For this review, take the finished solid that the model builds, in its own axes (mm). A direction names the side the tool comes from. Give positions to 0.01 mm unless a question says otherwise; leave off trailing zeros. Loops run counter-clockwise (first coordinate to the right, second up) from the corner with the lowest first, then second, coordinate; pieces in that order, holes last. Notation, with made-up numbers: (-15, 43.5) - (43, 43.5) arc R11 cw to (43, 52.5) - close; hole circle Ø4 at (-33.75, 12). An arc over 180 degrees is marked (long way). Put each result on its own line as item: value.
from build123d import *

# Parameters (mm, degrees)
BOSS_EXTRUDE1_START = -22799.561142
BOSS_EXTRUDE1_DEPTH = 600
CUT_EXTRUDE1_START  = 2846.116519
CUT_EXTRUDE1_DEPTH  = 541.072944
BOSS_EXTRUDE2_DEPTH = 498
CUT_EXTRUDE2_DEPTH  = 689.125788175


with BuildPart() as part:
    # Sketch3 → Boss-Extrude1 (new body)
    with BuildSketch(Plane(origin=(0, 0, 0), x_dir=(0, 0, -1), z_dir=(1, 0, 0)).offset(BOSS_EXTRUDE1_START)):
        Polygon((-40199.900195068, 2810.990103756), (-41009.724035702, 3620.813944389), (-41002.65296789, 3627.885012201), (-40199.900195068, 2825.132239379), align=None)
    extrude(amount=-BOSS_EXTRUDE1_DEPTH)

    # Sketch4 → Cut-Extrude1 (cut)
    with BuildSketch(Plane(origin=(0, 0, 0), x_dir=(1, 0, 0), z_dir=(0, 1, 0)).offset(CUT_EXTRUDE1_START)):
        with BuildLine():
            Line((-22799.561141737, -40360.17380628), (-23030.548097876, -40360.17380628))
            ThreePointArc((-23030.548097876, -40360.17380628), (-23093.121695819, -40297.600208337), (-23030.548097876, -40235.026610394))
            Line((-23030.548097876, -40235.026610394), (-22799.561141737, -40235.026610394))
            Line((-22799.561141737, -40235.026610394), (-22799.561141737, -40360.17380628))
        make_face()
        with BuildLine():
            Line((-22799.561141728, -40761.957418224), (-22897.41060103, -40761.957418224))
            ThreePointArc((-22897.41060103, -40761.957418224), (-22959.984198973, -40699.383820281), (-22897.41060103, -40636.810222338))
            Line((-22897.41060103, -40636.810222338), (-22799.561141728, -40636.810222338))
            Line((-22799.561141728, -40636.810222338), (-22799.561141728, -40761.957418224))
        make_face()
    extrude(amount=CUT_EXTRUDE1_DEPTH, mode=Mode.SUBTRACT)

    # Sketch5 → Boss-Extrude2 (add)
    with BuildSketch(Plane.ZY.offset(23399.561141728)):
        Polygon((40050.70934907, 2661.799257758), (40199.900195068, 2810.990103756), (40199.900195068, 2825.132239379), (40043.638281258, 2668.870325569), align=None)
    extrude(amount=-BOSS_EXTRUDE2_DEPTH)

    # Sketch6 → Cut-Extrude2 (cut, through all)
    with BuildSketch(Plane(origin=(0, -18687.383977844, 18687.383977844), x_dir=(1, 0, 0), z_dir=(0, 0.707106781, -0.707106781))):
        with BuildLine():
            Line((-23349.561141728, -30426.804477376), (-23164.561141728, -30426.804477376))
            ThreePointArc((-23164.561141728, -30426.804477376), (-23154.561141728, -30416.804477376), (-23164.561141728, -30406.804477376))
            Line((-23164.561141728, -30406.804477376), (-23359.561141728, -30406.804477376))
            ThreePointArc((-23359.561141728, -30406.804477376), (-23366.63220954, -30409.733409565), (-23369.561141728, -30416.804477376))
            Line((-23369.561141728, -30416.804477376), (-23369.561141728, -31160.804477376))
            ThreePointArc((-23369.561141728, -31160.804477376), (-23366.63220954, -31167.875545188), (-23359.561141728, -31170.804477376))
            Line((-23359.561141728, -31170.804477376), (-23039.561141728, -31170.804477376))
            ThreePointArc((-23039.561141728, -31170.804477376), (-23029.561141728, -31160.804477376), (-23039.561141728, -31150.804477376))
            Line((-23039.561141728, -31150.804477376), (-23349.561141728, -31150.804477376))
            Line((-23349.561141728, -31150.804477376), (-23349.561141728, -30990.804477376))
            Line((-23349.561141728, -30990.804477376), (-23039.561141728, -30990.804477376))
            ThreePointArc((-23039.561141728, -30990.804477376), (-23029.561141728, -30980.804477376), (-23039.561141728, -30970.804477376))
            Line((-23039.561141728, -30970.804477376), (-23349.561141728, -30970.804477376))
            Line((-23349.561141728, -30970.804477376), (-23349.561141728, -30606.804477376))
            Line((-23349.561141728, -30606.804477376), (-23164.561141728, -30606.804477376))
            ThreePointArc((-23164.561141728, -30606.804477376), (-23154.561141728, -30596.804477376), (-23164.561141728, -30586.804477376))
            Line((-23164.561141728, -30586.804477376), (-23349.561141728, -30586.804477376))
            Line((-23349.561141728, -30586.804477376), (-23349.561141728, -30426.804477376))
        make_face()
    extrude(amount=-CUT_EXTRUDE2_DEPTH, mode=Mode.SUBTRACT)


solid = part.part
1) Wall thickness on line 1 (Y direction, x = -23035.5, z = 40762); line 2 (Y direction, x = -23017.5, z = 40773); line 3 (Z direction, x = -23108.5, y = 3137): over which ranges is each line inside the solid? List them lowest first.
Geometry check:
line 1: y = 3373.09 to 3387.23
line 2: y = 3384.09 to 3398.23
line 3: z = 40511.77 to 40525.91
2) Take a section at D-D on z = 40489. State the section outline as (x, y) points.
Geometry check:
outline: (-23399.56, 3100.09) - (-23369.56, 3100.09) - (-23369.56, 3114.23) - (-23399.56, 3114.23) - close; (-23349.56, 3100.09) - (-22799.56, 3100.09) - (-22799.56, 3114.23) - (-23349.56, 3114.23) - close
3) For faces 1 (the face through (-22799.561, 2838, 40217)), 2 (the face through (-23349.561, 2881, 40263)), list the 3-axis set-ups (+Z, -Z, +X, -X, +Y, -Y) from which the entire face can be reached by the end or side of a thin tool; tool diameter is ignored.
Geometry check:
face 1: +Z, -Z, +X, +Y, -Y
face 2: +Z, -Z, +Y, -Y
4) Insertion check: pin 1 Ø1.5 at (x, y) = (-23217.5, 2993) entering from +Z; pin 2 Ø1.5 at (x, y) = (-22980.5, 2814.5) entering from +Z; pin 3 Ø10 at (x, y) = (-23105, 2926.5) entering from +Z. Each pin has a flat end and moves straight along its axis. Give the tip position at first contact, or say it passes through.
Geometry check:
pin 1: stops at z = 40382.66
pin 2: stops at z = 40204.16
pin 3: stops at z = 40320.41
5) Take a section at C-C on y = 3002. State the section outline as (x, z) points.
Geometry check:
outline: (-23399.56, 40376.77) - (-23369.56, 40376.77) - (-23369.56, 40390.91) - (-23399.56, 40390.91) - close; (-23349.56, 40376.77) - (-22799.56, 40376.77) - (-22799.56, 40390.91) - (-23349.56, 40390.91) - close
6) Take a section at A-A on x = -23136.5. State the section outline as (y, z) points, and give its area (3 significant figures).
Geometry check:
outline: (2661.8, 40050.71) - (2668.87, 40043.64) - (3212.28, 40587.05) - (3205.21, 40594.12) - close; (3219.35, 40608.26) - (3226.42, 40601.19) - (3339.56, 40714.33) - (3332.49, 40721.4) - close; (3346.63, 40735.54) - (3353.7, 40728.47) - (3627.89, 41002.65) - (3620.81, 41009.72) - close
area: 13,200 mm²
7) Take a section at B-B on x = -23275.5. State the section outline as (y, z) points.
Geometry check:
outline: (2661.8, 40050.71) - (2668.87, 40043.64) - (2813.47, 40188.24) - (2806.4, 40195.31) - close; (2820.54, 40209.45) - (2827.62, 40202.38) - (2940.75, 40315.52) - (2933.68, 40322.59) - close; (2947.82, 40336.73) - (2954.9, 40329.66) - (3212.28, 40587.05) - (3205.21, 40594.12) - close; (3219.35, 40608.26) - (3226.42, 40601.19) - (3339.56, 40714.33) - (3332.49, 40721.4) - close; (3346.63, 40735.54) - (3353.7, 40728.47) - (3627.89, 41002.65) - (3620.81, 41009.72) - close
